```python
from build123d import *

# Parameters (mm, degrees)
CHAMFER1_SIZE   = 6.062177826
CHAMFER1_SIZE_2 = 10.5


with BuildPart() as part:
    # Sketch2 → Revolve1 (revolve)
    with BuildSketch(Plane(origin=(0, 0, 0), x_dir=(1, 0, 0), z_dir=(0, 1, 0))):
        Polygon((1.5, 0), (3.85, 0), (3.85, 9), (9.75, 9), (9.75, 14), (3.85, 14), (3.85, 50), (1.5, 50), align=None)
    revolve(axis=Axis((0, 0, 0), (0, 0, -1)))

    # Chamfer1
    # the kernel refuses this chamfer: 10.5, 6.062177826 mm, written as the material it adds along each edge
    with BuildSketch(Plane(origin=(0, 0, -14), x_dir=(1, 0, 0), z_dir=(0, 1, 0))) as chamfer1_piece_1_section:
        Polygon((3.85 + CHAMFER1_SIZE, 0), (3.85, CHAMFER1_SIZE_2), (3.85, 0), align=None)
    chamfer1_piece_1 = revolve(axis=Axis((0, 0, -14), (0, 0, -1)), mode=Mode.PRIVATE)
    chamfer1_piece_1 = chamfer1_piece_1 & Plane(origin=(0, 0, -19.51769374), x_dir=(1, 0, 0), z_dir=(0, 0, -1)) * Cylinder(9.75, 42, mode=Mode.PRIVATE)
    add(chamfer1_piece_1)


solid = part.part
```
CAD build for the part. Positions are in the model's coordinates, mm. A direction names the side the tool comes from. Give positions to 0.01 mm unless a question says otherwise; leave off trailing zeros. Write each loop counter-clockwise with the first axis right and the second up, starting at its lowest first coordinate (ties: lowest second). Pieces come first, ordered by that corner, then holes. Notation, with made-up numbers: M -5.5,38.5 L 44.5,38.5 A23 cw 44.5,73.5 Z; hole C -21,-3.75 d11. An arc over 180 degrees is marked long. Return JSON: item names as keys, results as strings. Group by question number.
(1) Flat gauge pins, fed straight in: pin 1 Ø10 at (y, z) = (-3.5, -31.5) entering from +X; pin 2 Ø1.5 at (y, z) = (4, -7) entering from -X; pin 3 Ø1.5 at (x, z) = (3, -19.5) entering from -Y. Where does each tip first touch, or does it go through?
(2) Drill centre lines: L1, parallel to X at y = 0, z = -36; L2, parallel to Y at x = 0, z = -12.5. Where is each one in solid material? Low to high. Write a range as [from, to].
(3) Band-saw the part on C-C (z = -24). Give the cut face in (x, y).
(4) Band-saw the part on A-A (y = 0). Give the cut face in (x, z).
(5) Mould opens along X. For faces 1 (the face through (-4.2, -0.1, -9)), 2 (the face through (-0.83, 3.76, -4.56)), 3 (the face through (-1.5, -0.07, -24.65)) say: pulls with the +X half, pulls with the -X half, needs draft (parallel to the pull), parting line crosses it, or undercut.
(6) 3-axis set-ups, long thin cutter, end or side, ignore diameter. For faces 4 (the face through (-0.83, 3.76, -37.43)), 5 (the face through (-1.269, -9.667, -11.677)): which of +Z, -Z, +X, -X, +Y, -Y reach the whole face in a straight line?
Entries:
{
 "1": {"pin 1": "stops at x = 3.85", "pin 2": "stops at x = -2.06", "pin 3": "stops at y = -6.61"},
 "2": {"L1": "x = [-3.85, -1.5], [1.5, 3.85]", "L2": "y = [-9.75, -1.5], [1.5, 9.75]"},
 "3": {"outline": "C 0,0 d8.28; hole C 0,0 d3"},
 "4": {"outline": "M -9.75,-14.28 L -3.85,-24.5 L -3.85,-50 L -1.5,-50 L -1.5,0 L -3.85,0 L -3.85,-9 L -9.75,-9 Z; M 1.5,-50 L 3.85,-50 L 3.85,-24.5 L 9.75,-14.28 L 9.75,-9 L 3.85,-9 L 3.85,0 L 1.5,0 Z"},
 "5": {"face 1": "needs draft", "face 2": "parting line crosses it", "face 3": "undercut"},
 "6": {"face 4": "-Z", "face 5": "+Z, -Z"}
}
